Check sheet for the modelled part. Datum: model origin and axes. Units: mm. Give positions to 0.01 mm unless a question says otherwise; leave off trailing zeros. Order: outer loops, then holes, each group sorted by start corner. A loop starts at its lowest first (then second) coordinate and runs counter-clockwise, first axis right, second up. Notation, with made-up numbers: (0, 59) -> (22, 59) arc R11 cw to (22, 69) -> close; hole circle Ø9 at (-34.75, -26). An arc over 180 degrees is marked (long way). Write each question's results on one line, items separated by ' | '.
from build123d import *

# Parameters (mm, degrees)
BOSS_EXTRUDE1_DEPTH       = 22
M3X0_5_TAPPED_HOLE1_D     = 2.5
M3X0_5_TAPPED_HOLE1_DEPTH = 22


with BuildPart() as part:
    # Sketch1 → Boss-Extrude1 (new body)
    with BuildSketch(Plane(origin=(0, 0, 0), x_dir=(1, 0, 0), z_dir=(0, 1, 0))):
        Polygon((1.413165118, -2.517200366), (2.886542022, -0.034763291), (1.473376905, 2.482437075), (-1.413165118, 2.517200366), (-2.886542022, 0.034763291), (-1.473376905, -2.482437075), align=None)
    extrude(amount=BOSS_EXTRUDE1_DEPTH)

    # M3x0.5 Tapped Hole1
    with Locations(Plane(origin=(0, 22, 0), x_dir=(1, 0, 0), z_dir=(0, 1, 0))):
        with Locations((0, 0)):
            Hole(M3X0_5_TAPPED_HOLE1_D / 2, depth=M3X0_5_TAPPED_HOLE1_DEPTH)


solid = part.part
1. Mould release check, pull along X, two halves, no side actions. Record for faces 1 (the flat face through (-2.19, 10.85, 1.21)), 2 (the cylindrical face through (0.27, 10.85, 1.22)), 3 (the flat face through (1, 22, -1)), 4 (the flat face through (2.19, 10.85, -1.21)): +X half, -X half, draft (parallel to the pull), parting line (faces both ways), or undercut.
Verdict:
face 1: -X half | face 2: undercut | face 3: draft | face 4: +X half
2. Material ranges on probe 1 along X at (y, z) = (11.5, 0.05); probe 2 along X at (y, z) = (21, 0.15); probe 3 along Z at (x, y) = (0.1, 3.5), recorded low to high. Write a range as from..to.
Verdict:
probe 1: x = -2.84..-1.25, 1.25..2.88 | probe 2: x = -2.78..-1.24, 1.24..2.82 | probe 3: z = -2.5..-1.25, 1.25..2.5
3. Gauge pin test, flat ends, axial feed: pin 1 Ø1 at (y, z) = (17, 1) entering from -X; pin 2 Ø1.5 at (x, y) = (0, 10) entering from +Z; pin 3 Ø1 at (x, z) = (-0.5, -1) entering from +Y; pin 4 Ø2 at (y, z) = (7.5, 1) entering from -X. Record the tip position at first contact, or that the pin passes through.
Verdict:
pin 1: stops at x = -2.59 | pin 2: stops at z = 2.51 | pin 3: stops at y = 22 | pin 4: stops at x = -2.87
4. Section check A-A on x = -0.2. Record the cut outline in (y, z).
Verdict:
outline: (0, -2.5) -> (22, -2.5) -> (22, -1.23) -> (0, -1.23) -> close; (0, 1.23) -> (22, 1.23) -> (22, 2.5) -> (0, 2.5) -> close
5. Section check C-C on z = 1.05. Record the cut outline in (x, y), then the cut area to 3 significant figures.
Verdict:
outline: (-2.28, 0) -> (-0.68, 0) -> (-0.68, 22) -> (-2.28, 22) -> close; (0.68, 0) -> (2.28, 0) -> (2.28, 22) -> (0.68, 22) -> close | area: 70.5 mm^2
6. Section check B-B on y = 19.5. Record the cut outline in (x, z), then the cut area to 3 significant figures.
Verdict:
outline: (-2.89, -0.03) -> (-1.41, -2.52) -> (1.47, -2.48) -> (2.89, 0.03) -> (1.41, 2.52) -> (-1.47, 2.48) -> close; hole circle Ø2.5 at (0, 0) | area: 16.7 mm^2
7. Section check D-D on x = 2.2. Record the cut outline in (y, z), then the cut area to 3 significant figures.
Verdict:
outline: (0, -1.19) -> (22, -1.19) -> (22, 1.19) -> (0, 1.19) -> close | area: 52.4 mm^2
